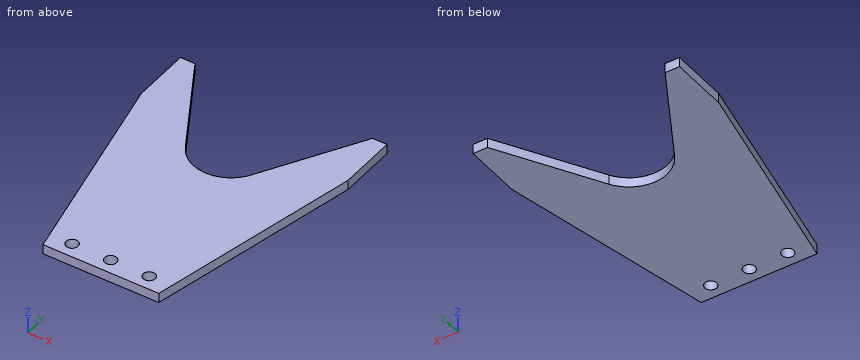
from build123d import *

# Parameters (mm, degrees)
BOSS_EXTRUDE1_DEPTH            = 6.35
F_5_16_0_3125_DIAMETER_HOLE1_D = 7.9375


with BuildPart() as part:
    # Sketch1 → Boss-Extrude1 (new body)
    with BuildSketch(Plane.XY):
        with BuildLine():
            Line((-21.667089577, -12.5095), (-58.438816897, 51.181))
            Line((-58.438816897, 51.181), (-67.963816897, 51.181))
            Line((-67.963816897, 51.181), (-67.963816897, 13.081))
            Line((-67.963816897, 13.081), (-38.1, -126.619))
            Line((-38.1, -126.619), (38.1, -126.619))
            Line((38.1, -126.619), (67.963816897, 13.081))
            Line((67.963816897, 13.081), (67.963816897, 51.181))
            Line((67.963816897, 51.181), (58.438816897, 51.181))
            Line((58.438816897, 51.181), (21.667089577, -12.5095))
            ThreePointArc((21.667089577, -12.5095), (0, -25.019), (-21.667089577, -12.5095))
        make_face()
    extrude(amount=BOSS_EXTRUDE1_DEPTH)

    # 5/16 (0.3125) Diameter Hole1 (through all)
    with Locations(Plane.XY.offset(6.35)):
        with Locations((-25.4, -117.094), (25.4, -117.094), (0, -117.094)):
            Hole(F_5_16_0_3125_DIAMETER_HOLE1_D / 2)


solid = part.part
Read the model definition and answer for the solid it produces. Units are mm, in the model's axes. Coordinates: 2 decimals unless noted, no trailing zeros. Loops run counter-clockwise (first coordinate to the right, second up) from the corner with the lowest first, then second, coordinate; pieces in that order, holes last. Notation, with made-up numbers: (24.5, 77.25) -> (41.5, 77.25) arc R26 ccw to (41.5, 115.25) -> close; hole circle Ø11 at (-15.5, 4). An arc over 180 degrees is marked (long way). Write item = value, one per line. Start each with the question number.
1) Find the intervals of material crossed by L1, parallel to Y at x = -25.4, z = 4.25; L2, parallel to Y at x = -28, z = 5; L3, parallel to X at y = -20, z = 2, in increasing order. Write a range as from..to.
2) The part is cut by section B-B, the plane z = 1.5. Determine the outline of the cut face in (x, y), plus the area to 3 significant figures.
3) The part is cut by section D-D, the plane y = -30. Determine the outline of the cut face in (x, z), plus the area to 3 significant figures.
4) The part is cut by section C-C, the plane x = 25.4. Determine the outline of the cut face in (y, z), plus the area to 3 significant figures.
5) Given P1, Ø2, axis at x = -52.5, z = 2, coming from the +Y side; P2, Ø6, axis at x = 34.5, y = -20, coming from the -Z side; P3, Ø3, axis at y = -63, z = 3, coming from the +X side; P4, Ø1, axis at y = -39, z = 5, coming from the +X side, each flat-ended and moving along its own axis, determine where each tip first touches the part or whether it passes through.
6) The part is cut by section A-A, the plane x = 0. Determine the outline of the cut face in (y, z).
Result:
q1.L1 = -126.62..-121.06, -113.13..-6.04
q1.L2 = -126.62..-120.09, -114.1..-1.54
q1.L3 = -60.89..-15.03, 15.03..60.89
q2.outline = (-67.96, 13.08) -> (-38.1, -126.62) -> (38.1, -126.62) -> (67.96, 13.08) -> (67.96, 51.18) -> (58.44, 51.18) -> (21.67, -12.51) arc R25.02 cw to (-21.67, -12.51) -> (-58.44, 51.18) -> (-67.96, 51.18) -> close; hole circle Ø7.94 at (-25.4, -117.09); hole circle Ø7.94 at (0, -117.09); hole circle Ø7.94 at (25.4, -117.09)
q2.area = 14,400 mm²
q3.outline = (-58.75, 0) -> (58.75, 0) -> (58.75, 6.35) -> (-58.75, 6.35) -> close
q3.area = 746 mm²
q4.outline = (-126.62, 0) -> (-121.06, 0) -> (-121.06, 6.35) -> (-126.62, 6.35) -> close; (-113.13, 0) -> (-6.04, 0) -> (-6.04, 6.35) -> (-113.13, 6.35) -> close
q4.area = 715 mm²
q5.P1 = 42.63
q5.P2 = 0
q5.P3 = 52.02
q5.P4 = 56.94
q6.outline = (-126.62, 0) -> (-121.06, 0) -> (-121.06, 6.35) -> (-126.62, 6.35) -> close; (-113.13, 0) -> (-25.02, 0) -> (-25.02, 6.35) -> (-113.13, 6.35) -> close
